```python
from build123d import *

# Parameters (mm, degrees)
SKETCH1_W           = 12.276797887
SKETCH1_H           = 46.74626888
BOSS_EXTRUDE1_DEPTH = 80
SKETCH8_W           = 46.74626888
SKETCH8_H           = 9.079638953
BOSS_EXTRUDE2_DEPTH = 10
CUT_EXTRUDE1_REACH  = 71.903
SKETCH10_R          = 5.704864585
FILLET1_R           = 2


with BuildPart() as part:
    # Sketch1 → Boss-Extrude1 (new body)
    with BuildSketch(Plane(origin=(0, 0, 0), x_dir=(1, 0, 0), z_dir=(0, 1, 0))):
        with Locations((-28.803256583, -3.777476273)):
            Rectangle(SKETCH1_W, SKETCH1_H)
    extrude(amount=BOSS_EXTRUDE1_DEPTH)

    # Sketch8 → Boss-Extrude2 (add)
    with BuildSketch(Plane(origin=(-22.664857639, 0, 0), x_dir=(0, 0, -1), z_dir=(1, 0, 0))):
        with Locations((-3.777476273, 49.574364566)):
            Rectangle(SKETCH8_W, SKETCH8_H)
    extrude(amount=BOSS_EXTRUDE2_DEPTH)

    # Sketch10 → Cut-Extrude1 (cut, up to next)
    with BuildSketch(Plane(origin=(0, 54.114184042, 0), x_dir=(1, 0, 0), z_dir=(0, 1, 0)), mode=Mode.PRIVATE) as cut_extrude1_sk1:
        with Locations((-12.664857639, -3.777476273)):
            Circle(SKETCH10_R)
    cut_extrude1_tool1 = extrude(cut_extrude1_sk1.sketch, amount=-CUT_EXTRUDE1_REACH, mode=Mode.PRIVATE) & part.part
    add(cut_extrude1_tool1.solids().sort_by_distance((-12.664858, 54.114184, 3.777476))[0], mode=Mode.SUBTRACT)

    # Fillet1
    fillet1_edges = [part.edges().sort_by_distance(p)[0] for p in [
        (-12.664857639, 49.574364566, -1.927388312),
        (-12.664857639, 49.574364566, 9.482340858),
    ]]
    fillet(fillet1_edges, radius=FILLET1_R)


solid = part.part
```
Verification items for the finished model (mm, model axes). A direction names the side the tool comes from. Give positions to 0.01 mm unless a question says otherwise; leave off trailing zeros. Order: outer loops, then holes, each group sorted by start corner. A loop starts at its lowest first (then second) coordinate and runs counter-clockwise, first axis right, second up. Notation, with made-up numbers: (13, -32) -> (62, -32) arc R11 cw to (62, -19) -> close; hole circle Ø10 at (-12, 19.25). An arc over 180 degrees is marked (long way). One line per item, written item: value.
(1) Tool access check on faces 1 (the face through (-19, 54.114, 4)), 2 (the face through (-12.665, 50, 19)), 3 (the face through (-13.067, 49.638, -2.461)), 4 (the face through (-19, 45.035, 4)). Record the directions out of +Z, -Z, +X, -X, +Y, -Y that give a thin tool (end or side, any length) a straight path to the whole face; none if there is none.
Final values:
face 1: +Z, -Z, +X, +Y
face 2: +Z, -Z, +X, +Y, -Y
face 3: +X, +Y, -Y
face 4: +Z, -Z, +X, -Y
(2) Gauge pin test, flat ends, axial feed: pin 1 (8 mm diameter, centred on y = 65.5, z = 12.5, fed in from +X); pin 2 (5 mm diameter, centred on x = -15.5, z = 10, fed in from +Y); pin 3 (6 mm diameter, centred on x = -19, y = 26, fed in from -Z). Record the tip position at first contact, or that the pin passes through.
Final values:
pin 1: x = -22.66
pin 2: y = 54.11
pin 3: through
(3) Scan lines: line 1 along X through (y, z) = (69.5, 20.5); line 2 along Y through (x, z) = (-22.5, 24); line 3 along X through (y, z) = (52.5, 5). Record each from-to range of solid material in increasing order. Write a range as [from, to].
Final values:
line 1: [-34.94, -22.66]
line 2: [45.03, 54.11]
line 3: [-34.94, -18.24]
(4) Sectioned sample at A-A on z = 16. Record the cut outline in (x, y).
Final values:
outline: (-34.94, 0) -> (-22.66, 0) -> (-22.66, 45.03) -> (-12.66, 45.03) -> (-12.66, 54.11) -> (-22.66, 54.11) -> (-22.66, 80) -> (-34.94, 80) -> close
(5) Sectioned sample at C-C on z = 8. Record the cut outline in (x, y).
Final values:
outline: (-34.94, 0) -> (-22.66, 0) -> (-22.66, 45.03) -> (-16.5, 45.03) -> (-16.5, 54.11) -> (-22.66, 54.11) -> (-22.66, 80) -> (-34.94, 80) -> close
(6) Draft check along Z on faces 5 (the face through (-29, 39, -19.596)), 6 (the face through (-13.067, 49.638, 10.016)), 7 (the face through (-34.942, 39, 4)). Enter one of: pulls with the +Z half, pulls with the -Z half, needs draft (parallel to the pull), parting line crosses it, or undercut.
Final values:
face 5: pulls with the -Z half
face 6: undercut
face 7: needs draft
(7) Sectioned sample at B-B on y = 28.5. Record the cut outline in (x, z).
Final values:
outline: (-34.94, -19.6) -> (-22.66, -19.6) -> (-22.66, 27.15) -> (-34.94, 27.15) -> close
